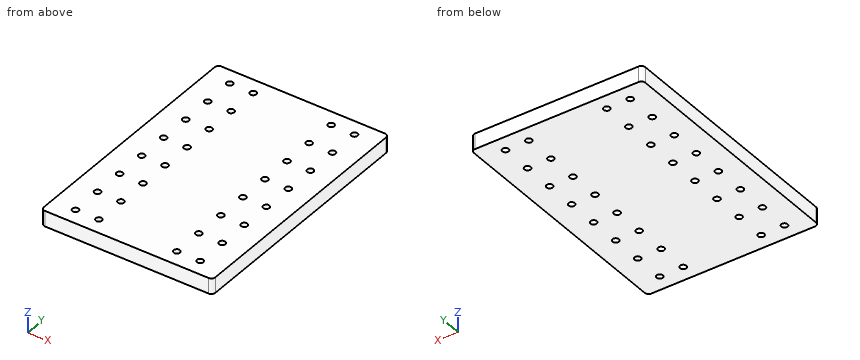
```python
from build123d import *

# Parameters (mm, degrees)
MODEL_W             = 139.7
MODEL_H             = 203.2
MODEL_R             = 2.5527
BOSS_EXTRUDE1_DEPTH = 12.7
FILLET1_R           = 3.175


with BuildPart() as part:
    # Model → Boss-Extrude1 (new body)
    with BuildSketch(Plane.XY):
        with Locations((540.658235294, 473.817647059)):
            Rectangle(MODEL_W, MODEL_H)
        with Locations((591.458235294, 562.717647059)):
            Circle(MODEL_R, mode=Mode.SUBTRACT)
        with Locations((591.458235294, 486.517647059)):
            Circle(MODEL_R, mode=Mode.SUBTRACT)
        with Locations((489.858235294, 486.517647059)):
            Circle(MODEL_R, mode=Mode.SUBTRACT)
        with Locations((489.858235294, 562.717647059)):
            Circle(MODEL_R, mode=Mode.SUBTRACT)
        with Locations((591.458235294, 537.317647059)):
            Circle(MODEL_R, mode=Mode.SUBTRACT)
        with Locations((489.858235294, 537.317647059)):
            Circle(MODEL_R, mode=Mode.SUBTRACT)
        with Locations((591.458235294, 511.917647059)):
            Circle(MODEL_R, mode=Mode.SUBTRACT)
        with Locations((489.858235294, 511.917647059)):
            Circle(MODEL_R, mode=Mode.SUBTRACT)
        with Locations((508.908235294, 486.517647059)):
            Circle(MODEL_R, mode=Mode.SUBTRACT)
        with Locations((508.908235294, 562.717647059)):
            Circle(MODEL_R, mode=Mode.SUBTRACT)
        with Locations((508.908235294, 537.317647059)):
            Circle(MODEL_R, mode=Mode.SUBTRACT)
        with Locations((508.908235294, 511.917647059)):
            Circle(MODEL_R, mode=Mode.SUBTRACT)
        with Locations((572.408235294, 562.717647059)):
            Circle(MODEL_R, mode=Mode.SUBTRACT)
        with Locations((572.408235294, 486.517647059)):
            Circle(MODEL_R, mode=Mode.SUBTRACT)
        with Locations((572.408235294, 537.317647059)):
            Circle(MODEL_R, mode=Mode.SUBTRACT)
        with Locations((572.408235294, 511.917647059)):
            Circle(MODEL_R, mode=Mode.SUBTRACT)
        with Locations((591.458235294, 410.317647059)):
            Circle(MODEL_R, mode=Mode.SUBTRACT)
        with Locations((489.858235294, 410.317647059)):
            Circle(MODEL_R, mode=Mode.SUBTRACT)
        with Locations((591.458235294, 435.717647059)):
            Circle(MODEL_R, mode=Mode.SUBTRACT)
        with Locations((489.858235294, 435.717647059)):
            Circle(MODEL_R, mode=Mode.SUBTRACT)
        with Locations((508.908235294, 410.317647059)):
            Circle(MODEL_R, mode=Mode.SUBTRACT)
        with Locations((508.908235294, 435.717647059)):
            Circle(MODEL_R, mode=Mode.SUBTRACT)
        with Locations((572.408235294, 410.317647059)):
            Circle(MODEL_R, mode=Mode.SUBTRACT)
        with Locations((572.408235294, 435.717647059)):
            Circle(MODEL_R, mode=Mode.SUBTRACT)
        with Locations((591.458235294, 384.917647059)):
            Circle(MODEL_R, mode=Mode.SUBTRACT)
        with Locations((489.858235294, 384.917647059)):
            Circle(MODEL_R, mode=Mode.SUBTRACT)
        with Locations((508.908235294, 384.917647059)):
            Circle(MODEL_R, mode=Mode.SUBTRACT)
        with Locations((572.408235294, 384.917647059)):
            Circle(MODEL_R, mode=Mode.SUBTRACT)
        with Locations((591.458235294, 461.117647059)):
            Circle(MODEL_R, mode=Mode.SUBTRACT)
        with Locations((489.858235294, 461.117647059)):
            Circle(MODEL_R, mode=Mode.SUBTRACT)
        with Locations((508.908235294, 461.117647059)):
            Circle(MODEL_R, mode=Mode.SUBTRACT)
        with Locations((572.408235294, 461.117647059)):
            Circle(MODEL_R, mode=Mode.SUBTRACT)
    extrude(amount=BOSS_EXTRUDE1_DEPTH)

    # Fillet1
    fillet1_edges = [part.edges().sort_by_distance(p)[0] for p in [
        (610.508235294, 372.217647059, 6.35),
        (470.808235294, 372.217647059, 6.35),
        (470.808235294, 575.417647059, 6.35),
        (610.508235294, 575.417647059, 6.35),
    ]]
    fillet(fillet1_edges, radius=FILLET1_R)


solid = part.part
```
Build history of the part. All positions in model axes, mm. Round coordinates to 2 decimals unless told otherwise and drop trailing zeros. Answer in a Markdown table with one row per item.
1) Pin check, flat tip, straight feed: P1, Ø3, axis at x = 591.46, y = 562.72, coming from the -Z side. Stop position of the tip, or through.
Values:
| item | result |
|---|---|
| P1 | through |
2) Band-saw the part on A-A on z = 3. Give the number of separate pieces and of enclosed holes in the cut face, and give its area (3 significant figures).
Values:
| item | result |
|---|---|
| separate pieces | 1 |
| enclosed holes | 32 |
| area | 27,700 mm2 |
3) Wall check: L1, parallel to X at y = 387, z = 3.5; L2, parallel to X at y = 408, z = 9. Give the ranges that are in metal, low to high.
Values:
| item | result |
|---|---|
| L1 | 470.81 to 488.38, 491.33 to 507.43, 510.38 to 570.93, 573.88 to 589.98, 592.93 to 610.51 |
| L2 | 470.81 to 488.79, 490.93 to 507.84, 509.98 to 571.34, 573.48 to 590.39, 592.53 to 610.51 |
